Can you work these out from the model? Positions are in its coordinate system, mm. A direction names the side the tool comes from. Round coordinates to 2 decimals unless told otherwise and drop trailing zeros. Write each loop counter-clockwise with the first axis right and the second up, starting at its lowest first coordinate (ties: lowest second). Pieces come first, ordered by that corner, then holes. Notation, with made-up numbers: (28, 68) - (50, 68) arc R28 ccw to (50, 102) - close; hole circle Ø8 at (67, -25.75). An arc over 180 degrees is marked (long way). One line per item, written item: value. Start each with the question number.
(1) I want a section at C-C on z = 5.25. List the corners of the cut face in (x, y) for me.
(2) I want a section at D-D on x = 0. List the corners of the cut face in (y, z) for me (3 decimals), plus the area to 3 significant figures.
(3) I want a section at A-A on y = 0. List the corners of the cut face in (x, z) for me.
(4) Thinking about a two-plate mould opening in X: for faces 1 (the face through (-24.93, -112.265, 9.367)), 2 (the face through (-84.5, -52.1, 14)), 3 (the face through (-1, 86, 0)), 4 (the face through (-67.453, -51.721, 9.367)), which applies, +X half, -X half, draft (parallel to the pull), parting line (faces both ways), or undercut?
(5) I'm going to push flat-ended pins straight in: pin 1 Ø6 at (y, z) = (47.5, 9) entering from -X; pin 2 Ø8 at (y, z) = (7, 14) entering from -X; pin 3 Ø3 at (x, y) = (-85, -51) entering from +Z. Where does each tip first touch, or does it pass through?
(6) I want a section at B-B on x = 31. List the corners of the cut face in (y, z) for me.
(7) On a 3-axis mill with a long thin cutter (end or side, diameter ignored), from which of +Z, -Z, +X, -X, +Y, -Y can I reach the whole of each face in a straight line? I mean faces 5 (the face through (-0.635, 104.834, 16.535)), 6 (the face through (-9, -85, 19)), 7 (the face through (3, 101, 2)). Say none if no direction works.
(8) If I drill on L1, parallel to Y at x = 0, z = 11.5; L2, parallel to X at y = -49.5, z = 8; L3, parallel to X at y = -50, z = 1, over which ranges is the centre line in solid material (lowest first)? Write a range as from..to.
from build123d import *

# Parameters (mm, degrees)
F0_R           = 115
F0_R_2         = 85
F1_DEPTH       = 19
F2_R           = 6
F3_DEPTH       = 2
F5_D           = 5.5
F5_CBORE_D     = 9.75
F5_CBORE_DEPTH = 5


with BuildPart() as f1:
    # F0 (on Top) → F1 (new body)
    with BuildSketch(Plane.XY):
        Circle(F0_R)
        Circle(F0_R_2, mode=Mode.SUBTRACT)
    extrude(amount=F1_DEPTH)

    # F2 (on face) → F3 (cut)
    with BuildSketch(Plane(origin=(0, 0, 0), x_dir=(1, 0, 0), z_dir=(0, 0, -1))):
        with Locations((0, -100)):
            Circle(F2_R)
        with Locations((86.6025403784, 50)):
            Circle(F2_R)
        with Locations((-86.6025403784, 50)):
            Circle(F2_R)
    extrude(amount=-F3_DEPTH, mode=Mode.SUBTRACT)

    # F5 (through all)
    with Locations(Plane.XY.offset(19)):
        with Locations((0, 100), (86.6025403784, -50), (-86.6025403784, -50)):
            CounterBoreHole(F5_D / 2, F5_CBORE_D / 2, F5_CBORE_DEPTH)


solid = f1.part
Established:
1. outline: circle Ø230 at (0, 0); hole circle Ø5.5 at (-86.6, -50); hole circle Ø170 at (0, 0); hole circle Ø5.5 at (0, 100); hole circle Ø5.5 at (86.6, -50)
2. outline: (-115, 0) - (-85, 0) - (-85, 19) - (-115, 19) - close; (85, 0) - (94, 0) - (94, 2) - (97.25, 2) - (97.25, 14) - (95.125, 14) - (95.125, 19) - (85, 19) - close; (102.75, 2) - (106, 2) - (106, 0) - (115, 0) - (115, 19) - (104.875, 19) - (104.875, 14) - (102.75, 14) - close
2. area: 1,000 mm2
3. outline: (-115, 0) - (-85, 0) - (-85, 19) - (-115, 19) - close; (85, 0) - (115, 0) - (115, 19) - (85, 19) - close
4. face 1: parting line
4. face 2: undercut
4. face 3: draft
4. face 4: undercut
5. pin 1: x = -106.04
5. pin 2: x = -114.96
5. pin 3: z = 14
6. outline: (-110.74, 0) - (-79.15, 0) - (-79.15, 19) - (-110.74, 19) - close; (79.15, 0) - (110.74, 0) - (110.74, 19) - (79.15, 19) - close
7. face 5: +Z
7. face 6: +Z, +X, -X, +Y, -Y
7. face 7: -Z
8. L1: -115..-85, 85..97.25, 102.75..115
8. L2: -103.8..-89.31, -83.9..-69.1, 69.1..83.9, 89.31..103.8
8. L3: -103.56..-92.6, -80.6..-68.74, 68.74..80.6, 92.6..103.56
